Autodesk Fusion 360 part; units mm, degrees
sketch "スケッチ1" plane through (0, 0, 0) normal (0, 0, 1) x (1, 0, 0)
  line L0 (0, 0) -> (60, 0)
  line L1 (60, 0) -> (60, 34)
  line L2 (60, 34) -> (0, 34)
  line L3 (0, 34) -> (0, 0)
  dimension "d1" = 60
  dimension "d2" = 34
extrude "押し出し1" add sketch "スケッチ1" along normal blind 10
sketch "スケッチ2" plane through (0, 0, 10) normal (0, 0, 1) x (-1, 0, 0)
  line L0 (0, -34) -> (0, 0)
  line L1 (0, 0) -> (-60, 0)
  line L2 (-60, 0) -> (-60, -34)
  line L3 (-60, -34) -> (0, -34)
  line L4 (-60, 0) -> (-58, 0)
  line L5 (-58, 0) -> (-58, -28)
  line L6 (-58, -28) -> (-60, -28)
  line L7 (-60, -28) -> (-60, 0)
  dimension "d5" = 2
  dimension "d6" = 28
extrude "押し出し2" cut sketch "スケッチ2" against normal blind 10 contours L1 L2 L4 L5 L6 L7
sketch "スケッチ3" plane through (0, 0, 10) normal (0, 0, 1) x (-1, 0, 0)
  line L0 (-58, 0) -> (-58, -28)
  line L1 (-58, -28) -> (-60, -28)
  line L2 (-60, -28) -> (-60, -34)
  line L3 (-60, -34) -> (0, -34)
  line L4 (0, -34) -> (0, 0)
  line L5 (0, 0) -> (-58, 0)
  line L6 (0, 0) -> (-2, 0)
  line L7 (-2, 0) -> (-2, -28)
  line L8 (-2, -28) -> (0, -28)
  line L9 (0, -28) -> (0, 0)
  dimension "d9" = 2
  dimension "d10" = 28
extrude "押し出し3" cut sketch "スケッチ3" against normal blind 15 contours L4 L5 L6 L7 L8 L9
sketch "スケッチ4" plane through (0, 0, 0) normal (0, 1, 0) x (1, 0, 0)
sketch "スケッチ5" plane through (0, 0, 0) normal (0, -1, 0) x (1, 0, 0)
  line L0 (2, 10) -> (2, 0)
  line L1 (2, 0) -> (58, 0)
  line L2 (58, 0) -> (58, 10)
  line L3 (58, 10) -> (2, 10)
  line L4 (58, 10) -> (2, 10)
  line L5 (2, 10) -> (2, 7)
  line L6 (2, 7) -> (58, 7)
  line L7 (58, 7) -> (58, 10)
  dimension "d13" = 3
extrude "押し出し4" cut sketch "スケッチ5" against normal blind 32 contours L0 L2 L3 L4 L5 L6 L7
sketch "スケッチ6" plane through (0, 0, 10) normal (0, 0, 1) x (-1, 0, 0)
  line L0 (-2, -28) -> (-2, -32)
  line L1 (-2, -32) -> (-58, -32)
  line L2 (-58, -32) -> (-58, -28)
  line L3 (-58, -28) -> (-60, -28)
  line L4 (-60, -28) -> (-60, -34)
  line L5 (-60, -34) -> (0, -34)
  line L6 (0, -34) -> (0, -28)
  line L7 (0, -28) -> (-2, -28)
  line L8 (-2, -28) -> (0, -28)
  line L9 (0, -28) -> (0, -32)
  line L10 (0, -32) -> (-2, -32)
  line L11 (-2, -32) -> (-2, -28)
extrude "押し出し5" cut sketch "スケッチ6" against normal blind 3 contours L0 L6 L7 L8 L9 L10 L11
sketch "スケッチ7" plane through (0, 0, 10) normal (0, 0, 1) x (-1, 0, 0)
  line L0 (0, -32) -> (-58, -32)
  line L1 (-58, -32) -> (-58, -28)
  line L2 (-58, -28) -> (-60, -28)
  line L3 (-60, -28) -> (-60, -34)
  line L4 (-60, -34) -> (0, -34)
  line L5 (0, -34) -> (0, -32)
  line L6 (-58, -32) -> (-60, -32)
  line L7 (-60, -32) -> (-60, -28)
  line L8 (-60, -28) -> (-58, -28)
  line L9 (-58, -28) -> (-58, -32)
extrude "押し出し6" cut sketch "スケッチ7" against normal blind 3 contours L1 L2 L3 L6 L7 L8 L9
sketch "スケッチ8" plane through (0, 0, 10) normal (0, 0, 1) x (-1, 0, 0)
  line L0 (-60, -32) -> (-60, -34)
  line L1 (-60, -34) -> (0, -34)
  line L2 (0, -34) -> (0, -32)
sketch "スケッチ9" plane through (0, 0, 10) normal (0, 0, 1) x (1, 0, 0)
sketch "スケッチ10" plane through (0, 32, 0) normal (0, -1, 0) x (1, 0, 0)
  line L0 (60, 10) -> (0, 10)
  line L1 (0, 10) -> (0, 7)
  line L2 (0, 7) -> (60, 7)
  line L3 (60, 7) -> (60, 10)
  spline S0 degree 5 poles (0, 7) (1.2, 7.2275) (3.6, 7.6628) (7.2, 8.256) (12, 8.9257) (18, 9.5472) (24, 9.9337) (30, 10.066) (36, 9.9337) (42, 9.5472) (48, 8.9257) (52.8, 8.256) (56.4, 7.6628) (58.8, 7.2275) (60, 7) knots 0 0 0 0 0 0 0.1 0.2 0.3 0.4 0.5 0.6 0.7 0.8 0.9 1 1 1 1 1 1
  point P0 (30, 10)
extrude "押し出し7" cut sketch "スケッチ10" against normal blind 16 contours L0 L3 S0 | L0 L1 S0
sketch "スケッチ11" plane through (0, 0, 0) normal (0, 0, -1) x (1, 0, 0)
  line L0 (2, -28) -> (0, -28)
  line L1 (0, -28) -> (0, -34)
  line L2 (0, -34) -> (60, -34)
  line L3 (60, -34) -> (60, -28)
  line L4 (60, -28) -> (58, -28)
  line L5 (58, -28) -> (58, 0)
  line L6 (58, 0) -> (2, 0)
  line L7 (2, 0) -> (2, -28)
Geometry: final body of the model. Coordinates: model frame, mm. A direction names the side the tool comes from. Round coordinates to 2 decimals unless told otherwise and drop trailing zeros. Loops run counter-clockwise (first coordinate to the right, second up) from the corner with the lowest first, then second, coordinate; pieces in that order, holes last. Notation, with made-up numbers: M -18.5,-11 L -10.5,-11 A12 cw -10.5,1 Z; hole C 30.5,87.25 d7. An arc over 180 degrees is marked long. Put each result on its own line as item: value. Start each with the question number.
(1) Section query B-B (y = 29). Return loops of the section in (x, z), then the cut area to 3 significant figures.
(2) Set-up query: faces 1 (the face through (1, 28, 4)), 2 (the face through (30, 16, 7)), 3 (the face through (30, 34, 5)), 4 (the face through (58, 14, 4)). Return all of +Z, -Z, +X, -X, +Y, -Y with unobstructed straight access to the full face (end or side cutting, diameter ignored); none if empty.
(3) Material intervals for line 1 along Z through (x, y) = (36.5, 9.5); line 2 along X through (y, z) = (7, 5.5); line 3 along Y through (x, z) = (20, 8.25), sorted ascending. Write a range as [from, to].
(4) Contact query for flat-ended pins moving along their axis: pin 1 Ø5.5 at (y, z) = (15, 3) entering from -X; pin 2 Ø4 at (x, y) = (44.5, 10.5) entering from +Z; pin 3 Ø1.5 at (x, z) = (38.5, 8) entering from -Y. Output: stop coordinate, or through.
(5) Section query A-A (z = 2.75). Return loops of the section in (x, y).
(6) Section query C-C (y = 2). Return loops of the section in (x, z), then the cut area to 3 significant figures.
Findings below:
1. outline: M 0,0 L 60,0 L 60,7 L 0,7 Z
1. area: 420 mm2
2. face 1: +Z, -Z, -X, -Y
2. face 2: +Z, +X, -X, -Y
2. face 3: +Z, -Z, +X, -X, +Y
2. face 4: +Z, -Z, +X, -Y
3. line 1: z = [0, 7]
3. line 2: x = [2, 58]
3. line 3: y = [32, 34]
4. pin 1: stops at x = 2
4. pin 2: stops at z = 7
4. pin 3: stops at y = 32
5. outline: M 0,28 L 2,28 L 2,0 L 58,0 L 58,28 L 60,28 L 60,34 L 0,34 Z
6. outline: M 2,0 L 58,0 L 58,7 L 2,7 Z
6. area: 392 mm2
